Geometry check sheet. Reference: the model listing, model coordinates, mm. Face numbers are marked on the shaded views. A direction names the side the tool comes from. Round coordinates to 2 decimals unless told otherwise and drop trailing zeros. Order: outer loops, then holes, each group sorted by start corner. A loop starts at its lowest first (then second) coordinate and runs counter-clockwise, first axis right, second up. Notation, with made-up numbers: (76, -25.5) - (85, -25.5) arc R22 cw to (85, -17.5) - close; hole circle Ø6 at (-1, -14). An arc over 180 degrees is marked (long way). Use a Markdown table: item, result. Add a question column.
(1) Thickness scan on line 1 along Y through (x, z) = (6, -5.25) (3 decimals); line 2 along Y through (x, z) = (28, -0.25); line 3 along X through (y, z) = (5, -3.25). Record the ranges inside material, lowest first. Write a range as [from, to].
(2) Mould release check, pull along Z, two halves, no side actions. Record for the marked faces 4, 5, 6 and 7: released by +Z, released by -Z, zero draft, split by the parting line, or undercut.
(3) Section check B-B on y = 6. Record the boundary of the cut face in (x, z), then the cut area to 3 significant figures.
(4) Section check C-C on y = 10.5. Give the number of separate pieces and of enclosed holes in the cut face, then the cut area to 3 significant figures.
(5) Gauge pin test, flat ends, axial feed: P1, Ø4.5, axis at x = 17, y = 3.5, coming from the -Z side; P2, Ø1.2, axis at y = 4.5, z = -3, coming from the +X side. Record the tip position at first contact, or that the pin passes through.
(6) Section check A-A on x = 25. Record the boundary of the cut face in (y, z) (3 decimals), then the cut area to 3 significant figures.
(7) Access from +Z, -Z, +X, -X, +Y, -Y to the whole of each face (thin tool, end or side, straight path). Record for the marked faces 1, 2 and 3.
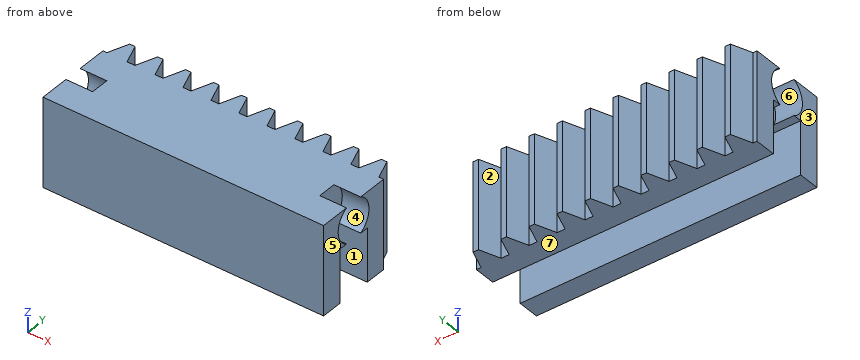
```python
from build123d import *

# Parameters (mm, degrees)
BLANKSKE_W              = 800
BLANKSKE_H              = 11
BLANK_DEPTH             = 10
TOOTHCUTSIM_DEPTH       = 801.138113078
TEETHCUTS_COUNT         = 255
TEETHCUTS_PITCH         = 3.14159265
CUT_EXTRUDE1_DEPTH      = 801.138113078
CUT_EXTRUDE1_DEPTH_BACK = 801.138113078
SKETCH1_W               = 6
SKETCH1_H               = 4
CUT_EXTRUDE2_DEPTH      = 801.138113078
CUT_EXTRUDE2_DEPTH_BACK = 801.138113078
SKETCH3_OUTSIDE_W       = 962.028
SKETCH3_OUTSIDE_H       = 173.028
SKETCH3_OUTSIDE_W_2     = 31.5
SKETCH3_OUTSIDE_H_2     = 25.836038267
CUT_EXTRUDE3_DEPTH      = 35.8317384
CUT_EXTRUDE3_DEPTH_BACK = 3
SKETCH4_R               = 2.25
CUT_EXTRUDE4_START      = -28.5
SKETCH4_2_R             = 2.25
CUT_EXTRUDE4_DEPTH      = 3


with BuildPart() as part:
    # BlankSke → Blank (new body)
    with BuildSketch(Plane.XY):
        with Locations((400, 5.5)):
            Rectangle(BLANKSKE_W, BLANKSKE_H)
    extrude(amount=-BLANK_DEPTH)

    # TooCutSkeSim → ToothCutSim (cut, through all)
    with BuildSketch(Plane.XY):
        Polygon((0.44443537, 8.75), (-0.44443537, 8.75), (-1.272613241, 11.0254), (1.272613241, 11.0254), align=None)
    toothcutsim = extrude(amount=-TOOTHCUTSIM_DEPTH, mode=Mode.SUBTRACT)

    # TeethCuts: ToothCutSim ×255
    with Locations(*[(i * TEETHCUTS_PITCH, 0, 0) for i in range(1, TEETHCUTS_COUNT)]):
        add(toothcutsim, mode=Mode.SUBTRACT)

    # Sketch1 → Cut-Extrude1 (cut, two sides: drawn at the far end of the back side and taken through both)
    with BuildSketch(Plane(origin=(800, 0, 0), x_dir=(0, 0, -1), z_dir=(1, 0, 0)).offset(-CUT_EXTRUDE1_DEPTH_BACK)):
        with Locations((7, 4.375)):
            Rectangle(SKETCH1_W, SKETCH1_H)
    extrude(amount=CUT_EXTRUDE1_DEPTH + CUT_EXTRUDE1_DEPTH_BACK, mode=Mode.SUBTRACT)

    # Sketch3 outside → Cut-Extrude2 (cut, two sides: drawn at the far end of the back side and taken through both)
    with BuildSketch(Plane.XY.offset(-CUT_EXTRUDE2_DEPTH_BACK)):
        with Locations((400, 5.5)):
            Rectangle(SKETCH3_OUTSIDE_W, SKETCH3_OUTSIDE_H)
        with Locations((15.75, 12.918019134)):
            Rectangle(SKETCH3_OUTSIDE_W_2, SKETCH3_OUTSIDE_H_2, mode=Mode.SUBTRACT)
    extrude(amount=CUT_EXTRUDE2_DEPTH + CUT_EXTRUDE2_DEPTH_BACK, mode=Mode.SUBTRACT)

    # Sketch4 → Cut-Extrude3 (cut, two sides: drawn at the far end of the back side and taken through both)
    with BuildSketch(Plane(origin=(31.5, 0, 0), x_dir=(0, 0, -1), z_dir=(1, 0, 0)).offset(-CUT_EXTRUDE3_DEPTH_BACK)):
        with Locations((2, 4.375)):
            Circle(SKETCH4_R)
    extrude(amount=CUT_EXTRUDE3_DEPTH + CUT_EXTRUDE3_DEPTH_BACK, mode=Mode.SUBTRACT)

    # Sketch4<2> → Cut-Extrude4 (cut)
    with BuildSketch(Plane(origin=(31.5, 0, 0), x_dir=(0, 0, -1), z_dir=(1, 0, 0)).offset(CUT_EXTRUDE4_START)):
        with Locations((2, 4.375)):
            Circle(SKETCH4_2_R)
    extrude(amount=-CUT_EXTRUDE4_DEPTH, mode=Mode.SUBTRACT)


solid = part.part
```
Check sheet entries:
| question | item | result |
|---|---|---|
| 1 | line 1 | y = [0, 2.375], [6.375, 8.75] |
| 1 | line 2 | y = [0, 8.75] |
| 1 | line 3 | x = [3, 28.5] |
| 2 | face 4 | undercut |
| 2 | face 5 | zero draft |
| 2 | face 6 | undercut |
| 2 | face 7 | released by -Z |
| 3 | outline | (0, -4) - (31.5, -4) - (31.5, -3.56) - (28.5, -3.56) - (28.5, -0.44) - (31.5, -0.44) - (31.5, 0) - (0, 0) - (0, -0.44) - (3, -0.44) - (3, -3.56) - (0, -3.56) - close |
| 3 | area | 107 mm2 |
| 4 | separate pieces | 10 |
| 4 | enclosed holes | 0 |
| 4 | area | 97.9 mm2 |
| 5 | P1 | stops at z = -10 |
| 5 | P2 | stops at x = 28.5 |
| 6 | outline | (0, -10) - (2.375, -10) - (2.375, -4) - (6.375, -4) - (6.375, -10) - (8.75, -10) - (8.75, 0) - (0, 0) - close |
| 6 | area | 63.5 mm2 |
| 7 | face 1 | -Z, +X, -X |
| 7 | face 2 | +Z, -Z, +Y |
| 7 | face 3 | +Z, -Z, -X, +Y, -Y |
